from build123d import *

# Parameters (mm, degrees)
F0_R     = 9.525
F1_DEPTH = 76.2
F2_W     = 11.43
F2_H     = 5.08
F3_DEPTH = 15.24
F5_R     = 2.15265
F6_DEPTH = 25.4
F7_R     = 4.2164
F8_DEPTH = 25.4


with BuildPart() as f1:
    # F0 (on Front) → F1 (new body)
    with BuildSketch(Plane.XZ):
        Circle(F0_R)
    extrude(amount=-F1_DEPTH)

    # F2 (on face) → F3 (cut)
    with BuildSketch(Plane(origin=(0, 76.2, 0), x_dir=(-1, 0, 0), z_dir=(0, 1, 0))):
        Rectangle(F2_W, F2_H)
    extrude(amount=-F3_DEPTH, mode=Mode.SUBTRACT)

    # F5 (on offset) → F6 (cut)
    with BuildSketch(Plane.XY.offset(9.525)):
        with Locations((0, 69.85)):
            Circle(F5_R)
    extrude(amount=-F6_DEPTH, mode=Mode.SUBTRACT)

    # F7 (on face) → F8 (cut)
    with BuildSketch(Plane.XZ):
        Circle(F7_R)
    extrude(amount=-F8_DEPTH, mode=Mode.SUBTRACT)


solid = f1.part
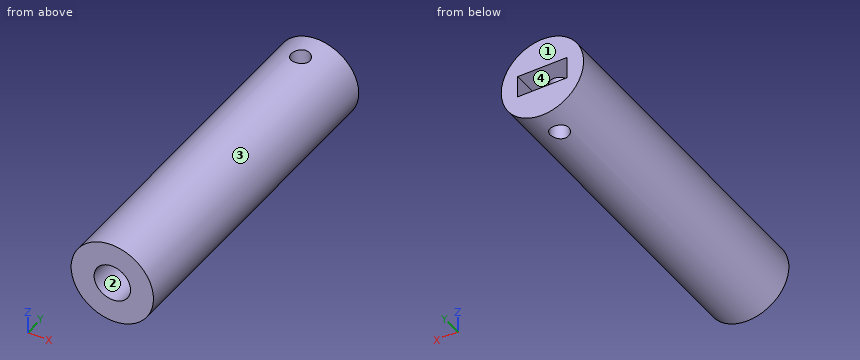
Verification items for the finished model (mm, model axes). Face numbers are marked on the shaded views. Coordinates: 2 decimals unless noted, no trailing zeros. Write each loop counter-clockwise with the first axis right and the second up, starting at its lowest first coordinate (ties: lowest second). Pieces come first, ordered by that corner, then holes. Notation, with made-up numbers: M 4.5,-25.75 L 19.5,-25.75 A29 cw 19.5,-0.75 Z; hole C 7.25,-8 d8. An arc over 180 degrees is marked long. Use CSV: the item, a comma, the result in double quotes.
Q1. Section check C-C, the plane z = 0. Enter the section's corners in (x, y) (3 decimals).
Computed values:
outline,"M -9.525,0 L -4.216,0 L -4.216,25.4 L 4.216,25.4 L 4.216,0 L 9.525,0 L 9.525,76.2 L 5.715,76.2 L 5.715,60.96 L -5.715,60.96 L -5.715,76.2 L -9.525,76.2 Z"
Q2. Section check D-D, the plane y = 55.5. Enter the section's corners in (x, z) (3 decimals).
Computed values:
outline,"C 0,0 d19.05"
Q3. Section check A-A, the plane x = 0. Enter the section's corners in (y, z) (3 decimals).
Computed values:
outline,"M 0,-9.525 L 67.697,-9.525 L 67.697,-2.54 L 60.96,-2.54 L 60.96,2.54 L 67.697,2.54 L 67.697,9.525 L 0,9.525 L 0,4.216 L 25.4,4.216 L 25.4,-4.216 L 0,-4.216 Z; M 72.003,-9.525 L 76.2,-9.525 L 76.2,-2.54 L 72.003,-2.54 Z; M 72.003,2.54 L 76.2,2.54 L 76.2,9.525 L 72.003,9.525 Z"
Q4. Go/stop test with flat-tipped pins: P1, Ø6.5, axis at x = 0, z = 0, coming from the -Y side; P2, Ø3, axis at x = -7, y = 20.5, coming from the -Z side; P3, Ø1, axis at x = -5.5, y = 21, coming from the +Z side. Record where each tip stops, or that it passes through.
Computed values:
P1,"y = 25.4"
P2,"z = -7.78"
P3,"z = 8.11"
Q5. Section check B-B, the plane y = 69.85. Enter the section's corners in (x, z) (3 decimals), and give its area (3 significant figures).
Computed values:
outline,"M -5.715,-2.54 L -5.715,2.54 L -2.153,2.54 L -2.153,9.279 A9.525 ccw -2.153,-9.279 L -2.153,-2.54 Z; M 2.153,-9.279 A9.525 ccw 2.153,9.279 L 2.153,2.54 L 5.715,2.54 L 5.715,-2.54 L 2.153,-2.54 Z"
area,"168 mm²"
Q6. Mould release check, pull along Z, two halves, no side actions. Record for the marked faces 1, 2, 3 and 4: pulls with the +Z half, pulls with the -Z half, needs draft (parallel to the pull), parting line crosses it, or undercut.
Computed values:
face 1,"needs draft"
face 2,"undercut"
face 3,"parting line crosses it"
face 4,"undercut"
Q7. Thickness scan on line 1 along Y through (x, z) = (0, 5); line 2 along Z through (x, y) = (0, 18.5) (3 decimals); line 3 along Y through (x, z) = (0, -0.75). Record the ranges inside material, lowest first. Write a range as [from, to].
Computed values:
line 1,"[0, 67.7], [72, 76.2]"
line 2,"[-9.525, -4.216], [4.216, 9.525]"
line 3,"[25.4, 60.96]"
